from build123d import *

# Parameters (mm, degrees)
SKETCH1_R                    = 4
BASE_FLANGE1_DEPTH           = 3.175
EDGE_FLANGE1_STRIP_W         = 14.1732
EDGE_FLANGE1_STRIP_H         = 3.175
EDGE_FLANGE1_STRIP_CUT_DEPTH = 18
EDGE_FLANGE1_DEPTH           = 18
EDGE_FLANGE2_STRIP_W         = 14.1732
EDGE_FLANGE2_STRIP_H         = 3.175
EDGE_FLANGE2_STRIP_CUT_DEPTH = 18
EDGE_FLANGE2_DEPTH           = 18
SKETCH12_R                   = 4.125
BOSS_EXTRUDE1_DEPTH          = 3.175


# Sheet-metal steps are written as plain solids
with BuildPart() as part:
    # Sketch1 → Base-Flange1 (new body)
    with BuildSketch(Plane(origin=(0, 0, 0), x_dir=(1, 0, 0), z_dir=(0, 1, 0))):
        with BuildLine():
            Line((-7, 12.5), (-7, 0))
            ThreePointArc((-7, 0), (-4.949747468, -4.949747468), (0, -7))
            Line((0, -7), (4, -7))
            ThreePointArc((4, -7), (8.949747468, -4.949747468), (11, 0))
            Line((11, 0), (11, 12.5))
            Line((11, 12.5), (-7, 12.5))
        make_face()
        with Locations(Location((0, 0, 0), (0, 0, 270))):
            Circle(SKETCH1_R, mode=Mode.SUBTRACT)
    extrude(amount=-BASE_FLANGE1_DEPTH)

    # Edge-Flange1 strip (across the edge) → Edge-Flange1 strip cut (cut)
    with BuildSketch(Plane(origin=(11, 0, -12.5), x_dir=(0, 0, 1), z_dir=(-1, 0, 0))):
        with Locations((-6.35, -1.5875)):
            Rectangle(EDGE_FLANGE1_STRIP_W, EDGE_FLANGE1_STRIP_H)
    extrude(amount=EDGE_FLANGE1_STRIP_CUT_DEPTH, mode=Mode.SUBTRACT)

    # Edge-Flange1 section (across the edge) → Edge-Flange1 (add)
    with BuildSketch(Plane(origin=(11, 0, -12.5), x_dir=(0, 0, 1), z_dir=(-1, 0, 0))):
        with BuildLine():
            Line((-3.175, 0.7366), (-3.175, 41.8875))
            Line((-3.175, 41.8875), (0, 41.8875))
            Line((0, 41.8875), (0, 0.7366))
            ThreePointArc((0, 0.7366), (0.215745145, 0.215745145), (0.7366, 0))
            Line((0.7366, 0), (0.7366, -3.175))
            ThreePointArc((0.7366, -3.175), (-2.029318885, -2.029318885), (-3.175, 0.7366))
        make_face()
    extrude(amount=EDGE_FLANGE1_DEPTH)

    # Edge-Flange2 strip (across the edge) → Edge-Flange2 strip cut (cut)
    with BuildSketch(Plane(origin=(-7, 41.8875, -15.675), x_dir=(0, -1, 0), z_dir=(1, 0, 0))):
        with Locations((-6.35, -1.5875)):
            Rectangle(EDGE_FLANGE2_STRIP_W, EDGE_FLANGE2_STRIP_H)
    extrude(amount=EDGE_FLANGE2_STRIP_CUT_DEPTH, mode=Mode.SUBTRACT)

    # Edge-Flange2 section (across the edge) → Edge-Flange2 (add)
    with BuildSketch(Plane(origin=(-7, 41.8875, -15.675), x_dir=(0, -1, 0), z_dir=(1, 0, 0))):
        with BuildLine():
            Line((-3.175, 0.7366), (-3.175, 3))
            Line((-3.175, 3), (0, 3))
            Line((0, 3), (0, 0.7366))
            ThreePointArc((0, 0.7366), (0.215745145, 0.215745145), (0.7366, 0))
            Line((0.7366, 0), (0.7366, -3.175))
            ThreePointArc((0.7366, -3.175), (-2.029318885, -2.029318885), (-3.175, 0.7366))
        make_face()
    extrude(amount=EDGE_FLANGE2_DEPTH)

    # Sketch12 → Boss-Extrude1 (add)
    with BuildSketch(Plane(origin=(0, 45.0625, 0), x_dir=(1, 0, 0), z_dir=(0, 1, 0))):
        with BuildLine():
            Line((11, 18.675), (-7, 18.675))
            ThreePointArc((-7, 18.675), (-5.730267968, 26.179894377), (-2.062407049, 32.849411251))
            Line((-2.062407049, 32.849411251), (26.4814048, 68.848399382))
            ThreePointArc((26.4814048, 68.848399382), (31.832032475, 71.825161968), (37.720386598, 70.146585866))
            Line((37.720386598, 70.146585866), (39.287532633, 68.903986451))
            ThreePointArc((39.287532633, 68.903986451), (42.264295219, 63.553358776), (40.585719117, 57.665004653))
            Line((40.585719117, 57.665004653), (12.041907268, 21.666016522))
            ThreePointArc((12.041907268, 21.666016522), (11.267932785, 20.258646945), (11, 18.675))
        make_face()
        with Locations(Location((32.749988941, 63.878001725, 0), (0, 0, 270))):
            Circle(SKETCH12_R, mode=Mode.SUBTRACT)
    extrude(amount=-BOSS_EXTRUDE1_DEPTH)


solid = part.part
Could you check a few things on this model? Use its own coordinates, in mm. A direction names the side the tool comes from. Give positions to 0.01 mm unless a question says otherwise; leave off trailing zeros. Order: outer loops, then holes, each group sorted by start corner. A loop starts at its lowest first (then second) coordinate and runs counter-clockwise, first axis right, second up. Notation, with made-up numbers: (-10.5, -18) -> (42.5, -18) arc R22 cw to (42.5, 17) -> close; hole circle Ø3 at (1, 65). An arc over 180 degrees is marked (long way). Answer in a Markdown table with one row per item. Add a question column.
Item 1: For faces 5 (the cylindrical face through (8.9, -1.6, 5)), 6 (the flat face through (2, 21, -12.5)), 7 (the flat face through (2, 21, -15.675)), which set-ups out of +Z, -Z, +X, -X, +Y, -Y let a thin tool reach every point of the face, with its end or its side?
Item 2: Please list where these lines run through material, in increasing order: probe 1 along X at (y, z) = (-1.4, 0); probe 2 along Y at (x, z) = (1.5, -8.5) (3 decimals); probe 3 along Z at (x, y) = (-2, 35.5) (3 decimals).
Item 3: Imagine slicing it at C-C (z = -8.5). List the corners of the cut face in (x, y) for me (3 decimals).
Item 4: Imagine slicing it at B-B (y = 5). List the corners of the cut face in (x, z) for me (3 decimals), and give its area (4 significant figures).
Item 5: I'm going to push flat-ended pins straight in: P1, Ø5.5, axis at x = 3.5, z = 0.5, coming from the +Y side; P2, Ø12, axis at y = 21, z = -4, coming from the -X side; P3, Ø5.5, axis at x = 5, y = 30, coming from the -Z side (3 decimals); P4, Ø12, axis at x = 9.5, z = -20.5, coming from the -Y side. Where does each tip first touch, or does it pass through?
Item 6: We'd pull the mould along Z, two halves only. Please class faces 1 (the cylindrical face through (1.87, 43.89, -13.62)), 2 (the flat face through (18, 41.888, -45)), 3 (the cylindrical face through (42.254, 43.497, -63.641)), 4 (the cylindrical face through (-3.905, -1.565, -0.867)): pulls with the +Z half, pulls with the -Z half, needs draft (parallel to the pull), parting line crosses it, or undercut.
Item 7: Imagine slicing it at A-A (z = 1). List the corners of the cut face in (x, y) for me (3 decimals).
Result:
| question | item | result |
|---|---|---|
| 1 | face 5 | +Z, +X, +Y, -Y |
| 1 | face 6 | +Z, +X, -X, +Y |
| 1 | face 7 | -Z, +X, -X, -Y |
| 2 | probe 1 | -7 to -4, 4 to 11 |
| 2 | probe 2 | -3.175 to 0 |
| 2 | probe 3 | -15.675 to -12.5 |
| 3 | outline | (-7, -3.175) -> (11, -3.175) -> (11, 0) -> (-7, 0) -> close |
| 4 | outline | (-7, -15.675) -> (11, -15.675) -> (11, -12.5) -> (-7, -12.5) -> close |
| 4 | area | 57.15 mm2 |
| 5 | P1 | y = 0 |
| 5 | P2 | through |
| 5 | P3 | z = -15.675 |
| 5 | P4 | y = -2.06 |
| 6 | face 1 | pulls with the +Z half |
| 6 | face 2 | needs draft |
| 6 | face 3 | parting line crosses it |
| 6 | face 4 | undercut |
| 7 | outline | (-6.928, -3.175) -> (-3.873, -3.175) -> (-3.873, 0) -> (-6.928, 0) -> close; (3.873, -3.175) -> (10.928, -3.175) -> (10.928, 0) -> (3.873, 0) -> close |
